Verification items for the finished model (mm, model axes). Round coordinates to 2 decimals unless told otherwise and drop trailing zeros. Loops run counter-clockwise (first coordinate to the right, second up) from the corner with the lowest first, then second, coordinate; pieces in that order, holes last. Notation, with made-up numbers: (-37, -31.75) -> (12, -31.75) arc R18 ccw to (12, -14.75) -> close; hole circle Ø6 at (48, 47.25). An arc over 180 degrees is marked (long way). Use a Markdown table: item, result. Add a question column.
```python
from build123d import *

# Parameters (mm, degrees)
F0_W     = 10
F0_H     = 12
F1_DEPTH = 10
F2_R     = 10
F3_R     = 5
F4_R     = 1
F5_R     = 0.79999
F6_R     = 0.5


# Not quite as in the source:
# - a fillet or chamfer is up to 0.001 mm smaller than in the source, because OpenCascade refuses the exact size
# - a feature names something its author has since deleted; it is built from what else it names


with BuildPart() as f1:
    # F0 (on Front) → F1 (new body, symmetric)
    with BuildSketch(Plane.XZ):
        Polygon((-0.8, 10), (-4.8, 10), (-10, -2), (0, -2), (0, 0), (-0.8, 0), align=None)
        Polygon((0, 0), (0, -2), (10, -2), (4.8, 10), (0.8, 10), (0.8, 0), align=None)
        with Locations((-5, -8)):
            Rectangle(F0_W, F0_H)
        with Locations((5, -8)):
            Rectangle(F0_W, F0_H)
    extrude(amount=F1_DEPTH, both=True)

    # F2
    f2_edges = [f1.edges().sort_by_distance(p)[0] for p in [
        (10, 0, -2),
        (-10, 0, -2),
    ]]
    fillet(f2_edges, radius=F2_R)

    # F3
    f3_edges = [f1.edges().sort_by_distance(p)[0] for p in [
        (4.8, 0, 10),
        (-4.8, 0, 10),
    ]]
    fillet(f3_edges, radius=F3_R)

    # F4
    f4_edges = [f1.edges().sort_by_distance(p)[0] for p in [
        (7.64037, 10, 3.4453),
        (7.64037, -10, 3.4453),
        (-7.64037, 10, 3.4453),
        (-7.64037, -10, 3.4453),
    ]]
    fillet(f4_edges, radius=F4_R)

    # F5 (radius 0.8 in the source; OpenCascade refuses exactly that, so slightly less here)
    f5_edges = [f1.edges().sort_by_distance(p)[0] for p in [
        (-0.8, 0, 0),
        (0.8, 0, 0),
    ]]
    fillet(f5_edges, radius=F5_R)

    # F6
    f6_edges = [f1.edges().sort_by_distance(p)[0] for p in [
        (-10, 0, -14),
        (-9.707107, 9.707107, -14),
        (-9.707107, -9.707107, -14),
        (0, 10, -14),
        (0, -10, -14),
        (9.707107, 9.707107, -14),
        (9.707107, -9.707107, -14),
        (10, 0, -14),
    ]]
    fillet(f6_edges, radius=F6_R)


solid = f1.part
```
1) Release check for a two-part mould opening along X. For faces 1 (the face through (-0.8, 0, 5)), 2 (the face through (7.36, -9.7, 3.38)), 3 (the face through (0.8, 0, 5)), 4 (the face through (-1.164, -9.715, 9.699)) record: released by +X, released by -X, zero draft, split by the parting line, or undercut.
2) Sectioned sample at B-B on x = -0.5. Enter the section's corners in (y, z), then the cut area to 3 significant figures.
3) Thickness scan on line 1 (X direction, y = 4.75, z = 7); line 2 (X direction, y = 7, z = 1); line 3 (Z direction, x = -1.75, y = 7.25). Record the ranges inside material, lowest first.
4) Go/stop test with flat-tipped pins: pin 1 (3 mm diameter, centred on x = 8, y = 5, fed in from +Z); pin 2 (4.5 mm diameter, centred on y = 0, z = 4, fed in from -X) (3 decimals); pin 3 (3 mm diameter, centred on y = -1.5, z = 7, fed in from +X); pin 4 (4 mm diameter, centred on x = -0.5, z = 4.5, fed in from -Y). Record where each tip stops, or that it passes through.
Geometry results:
| question | item | result |
|---|---|---|
| 1 | face 1 | undercut |
| 1 | face 2 | released by +X |
| 1 | face 3 | undercut |
| 1 | face 4 | zero draft |
| 2 | outline | (-10, -13.5) arc R0.5 ccw to (-9.5, -14) -> (9.5, -14) arc R0.5 ccw to (10, -13.5) -> (10, 0.18) -> (-10, 0.18) -> close |
| 2 | area | 283 mm^2 |
| 3 | line 1 | -6.1 to -0.8, 0.8 to 6.1 |
| 3 | line 2 | -8.7 to -0.8, 0.8 to 8.7 |
| 3 | line 3 | -14 to 9.99 |
| 4 | pin 1 | z = 6.08 |
| 4 | pin 2 | x = -8.375 |
| 4 | pin 3 | x = 6.75 |
| 4 | pin 4 | y = -10 |
